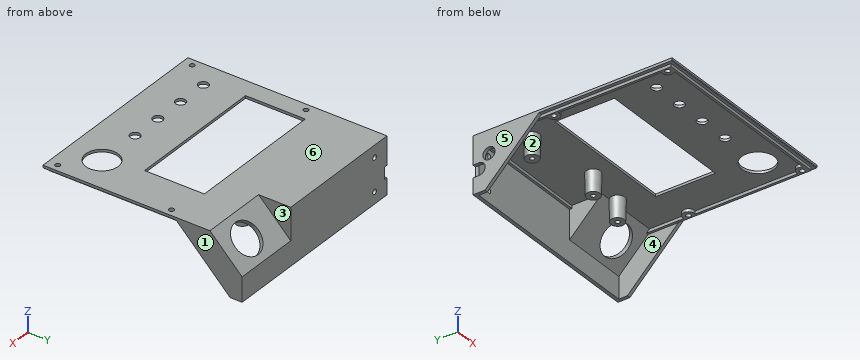
from build123d import *

# Parameters (mm, degrees)
CROQUIS1_W               = 140
CROQUIS1_H               = 140
FRENTE_DEPTH             = 1.8
CROQUIS32_W              = 135.2
CROQUIS32_H              = 135.2
CROQUIS32_W_2            = 132
CROQUIS32_H_2            = 132
SALIENTE_EXTRUIR5_DEPTH  = 2.1
SALIENTE_EXTRUIR6_DEPTH  = 2.1
VISERA_DEPTH             = 38
CORTAR_EXTRUIR1_DEPTH    = 2.4
SALIENTE_EXTRUIR9_DEPTH  = 50
CORTAR_EXTRUIR4_DEPTH    = 47
O_PE_REACH               = 113.138
CROQUIS39_R              = 11.25
CROQUIS15_R              = 1.75
ROSCA_DEPTH              = 3.9
MATRIZL1_COUNT           = 2
MATRIZL1_PITCH           = 80
MATRIZL1_COPY_1_DEPTH    = 2.1
MATRIZL1_COPY_2_SKETCH_R = 1.75
MATRIZL1_COPY_2_DEPTH    = 3.9
VISTA_DISPLAY_REACH      = 3.8
CROQUIS19_W              = 97.6
CROQUIS19_H              = 42
CROQUIS24_R              = 3.5
POTENCIOMETROS_DEPTH     = 1.8
MATRIZL3_COUNT           = 4
MATRIZL3_PITCH           = 22
CORTAR_EXTRUIR2_REACH    = 3.8
CROQUIS36_R              = 11.4
CHAFL_N1_SIZE            = 0.4
MPX_MOUNT_REACH          = 142
CROQUIS40_R              = 1.8
CROQUIS41_R              = 4.3
MPX_TUBBING_DEPTH        = 2.4
CROQUIS210_R             = 5
CROQUIS210_R_2           = 1.2
MEGA_UNO1_DEPTH          = 15
MEGA_UNO1_TAPER          = 1.5


with BuildPart() as part:
    # Croquis1 → FRENTE (new body)
    with BuildSketch(Plane.XY):
        Rectangle(CROQUIS1_W, CROQUIS1_H)
    extrude(amount=FRENTE_DEPTH)

    # Croquis32 → Saliente-Extruir5 (add)
    with BuildSketch(Plane(origin=(0, 0, 0), x_dir=(-1, 0, 0), z_dir=(0, 0, -1))):
        Rectangle(CROQUIS32_W, CROQUIS32_H)
        Rectangle(CROQUIS32_W_2, CROQUIS32_H_2, mode=Mode.SUBTRACT)
    extrude(amount=SALIENTE_EXTRUIR5_DEPTH)

    # Croquis33 → Saliente-Extruir6 (add)
    with BuildSketch(Plane(origin=(0, 0, 0), x_dir=(-1, 0, 0), z_dir=(0, 0, -1))):
        with BuildLine():
            Line((-67.6, -60.260263169), (-67.6, -66.339736831))
            ThreePointArc((-67.6, -66.339736831), (-61, -63.3), (-67.6, -60.260263169))
        make_face()
    saliente_extruir6 = extrude(amount=SALIENTE_EXTRUIR6_DEPTH)

    # Croquis29 → VISERA (add)
    with BuildSketch(Plane(origin=(0, 0, 0), x_dir=(-1, 0, 0), z_dir=(0, 0, -1))):
        Polygon((-70, 23.6), (-70, 70), (0, 70), (0, 67.6), (-67.6, 67.6), (-67.6, 23.6), align=None)
    visera = extrude(amount=VISERA_DEPTH)

    # Croquis30 → Cortar-Extruir1 (cut)
    with BuildSketch(Plane(origin=(70, 0, 0), x_dir=(0, 0, -1), z_dir=(1, 0, 0))):
        Polygon((0, 23.6), (38, 23.6), (38, 61.6), align=None)
    cortar_extruir1 = extrude(amount=-CORTAR_EXTRUIR1_DEPTH, mode=Mode.SUBTRACT)

    # Simetría3: VISERA, Cortar-Extruir1 across plane
    add(visera.mirror(Plane(origin=(0, 0, 0), x_dir=(0, 0, 1), z_dir=(1, 0, 0))))
    add(cortar_extruir1.mirror(Plane(origin=(0, 0, 0), x_dir=(0, 0, 1), z_dir=(1, 0, 0))), mode=Mode.SUBTRACT)

    # Croquis37 → Saliente-Extruir9 (add)
    with BuildSketch(Plane(origin=(70, 0, 0), x_dir=(0, 0, -1), z_dir=(1, 0, 0))):
        Polygon((25.070057685, 70), (-1.8, 43.129942315), (-1.8, 70), align=None)
    extrude(amount=-SALIENTE_EXTRUIR9_DEPTH)

    # Croquis38 → Cortar-Extruir4 (cut)
    with BuildSketch(Plane(origin=(70, 0, 0), x_dir=(0, 0, -1), z_dir=(1, 0, 0))):
        Polygon((20.827416998, 70), (-1.8, 47.372583002), (-1.8, 70), align=None)
    extrude(amount=-CORTAR_EXTRUIR4_DEPTH, mode=Mode.SUBTRACT)

    # Croquis39 → O-PE (cut, up to next)
    with BuildSketch(Plane(origin=(0, 24.586291501, 24.586291501), x_dir=(1, 0, 0), z_dir=(0, 0.707106781, 0.707106781)), mode=Mode.PRIVATE) as o_pe_sk1:
        with Locations((50, 48.224682477)):
            Circle(CROQUIS39_R)
    o_pe_tool1 = extrude(o_pe_sk1.sketch, amount=-O_PE_REACH, mode=Mode.PRIVATE) & part.part
    add(o_pe_tool1.solids().sort_by_distance((50, 58.686292, -9.513708))[0], mode=Mode.SUBTRACT)

    # Croquis15 → ROSCA (cut)
    with BuildSketch(Plane.XY.offset(1.8)):
        with Locations((65, -63.3)):
            Circle(CROQUIS15_R)
    rosca = extrude(amount=-ROSCA_DEPTH, mode=Mode.SUBTRACT)

    # Simetría4: Saliente-Extruir6, ROSCA across plane
    add(saliente_extruir6.mirror(Plane(origin=(0, 0, 0), x_dir=(0, 0, 1), z_dir=(1, 0, 0))))
    add(rosca.mirror(Plane(origin=(0, 0, 0), x_dir=(0, 0, 1), z_dir=(1, 0, 0))), mode=Mode.SUBTRACT)

    # MatrizL1: Saliente-Extruir6, ROSCA ×2
    with Locations(*[(0, i * MATRIZL1_PITCH, 0) for i in range(1, MATRIZL1_COUNT)]):
        add(saliente_extruir6)
        add(rosca, mode=Mode.SUBTRACT)

    # MatrizL1 copy 1 sketch → MatrizL1 copy 1 (add)
    with BuildSketch(Plane(origin=(0, 80, 0), x_dir=(1, 0, 0), z_dir=(0, 0, -1))):
        with BuildLine():
            Line((-67.6, 60.260263169), (-67.6, 66.339736831))
            ThreePointArc((-67.6, 66.339736831), (-61, 63.3), (-67.6, 60.260263169))
        make_face()
    extrude(amount=MATRIZL1_COPY_1_DEPTH)

    # MatrizL1 copy 2 sketch → MatrizL1 copy 2 (cut)
    with BuildSketch(Plane(origin=(0, 80, 1.8), x_dir=(-1, 0, 0), z_dir=(0, 0, 1))):
        with Locations((65, 63.3)):
            Circle(MATRIZL1_COPY_2_SKETCH_R)
    extrude(amount=-MATRIZL1_COPY_2_DEPTH, mode=Mode.SUBTRACT)

    # Croquis19 → VISTA-DISPLAY (cut, up to next)
    with BuildSketch(Plane(origin=(0, 0, 0), x_dir=(-1, 0, 0), z_dir=(0, 0, -1)), mode=Mode.PRIVATE) as vista_display_sk1:
        with Locations((8.2, 1)):
            Rectangle(CROQUIS19_W, CROQUIS19_H)
    vista_display_tool1 = extrude(vista_display_sk1.sketch, amount=-VISTA_DISPLAY_REACH, mode=Mode.PRIVATE) & part.part
    add(vista_display_tool1.solids().sort_by_distance((-8.2, 1, 0))[0], mode=Mode.SUBTRACT)

    # Croquis24 → POTENCIOMETROS (cut)
    with BuildSketch(Plane.XY.offset(1.8)):
        with Locations((-52, -46)):
            Circle(CROQUIS24_R)
    potenciometros = extrude(amount=-POTENCIOMETROS_DEPTH, mode=Mode.SUBTRACT)

    # MatrizL3: POTENCIOMETROS ×4
    with Locations(*[(i * MATRIZL3_PITCH, 0, 0) for i in range(1, MATRIZL3_COUNT)]):
        add(potenciometros, mode=Mode.SUBTRACT)

    # Croquis36 → Cortar-Extruir2 (cut, up to next)
    with BuildSketch(Plane(origin=(0, 0, 0), x_dir=(-1, 0, 0), z_dir=(0, 0, -1)), mode=Mode.PRIVATE) as cortar_extruir2_sk1:
        with Locations((-46, -46)):
            Circle(CROQUIS36_R)
    cortar_extruir2_tool1 = extrude(cortar_extruir2_sk1.sketch, amount=-CORTAR_EXTRUIR2_REACH, mode=Mode.PRIVATE) & part.part
    add(cortar_extruir2_tool1.solids().sort_by_distance((46, -46, 0))[0], mode=Mode.SUBTRACT)

    # Chaflán1
    chafl_n1_edges = [part.edges().sort_by_distance(p)[0] for p in [
        (0, -70, 0),
    ]]
    chamfer(chafl_n1_edges, length=CHAFL_N1_SIZE)

    # Croquis40 → MPX-MOUNT (cut, up to next)
    with BuildSketch(Plane(origin=(0, 70, 0), x_dir=(1, 0, 0), z_dir=(0, 1, 0)), mode=Mode.PRIVATE) as mpx_mount_sk1:
        with Locations((-58, 29.75)):
            Circle(CROQUIS40_R)
    mpx_mount_tool1 = extrude(mpx_mount_sk1.sketch, amount=-MPX_MOUNT_REACH, mode=Mode.PRIVATE) & part.part
    add(mpx_mount_tool1.solids().sort_by_distance((-58, 70, -29.75))[0], mode=Mode.SUBTRACT)
    # Croquis40 → MPX-MOUNT (cut, up to next)
    with BuildSketch(Plane(origin=(0, 70, 0), x_dir=(1, 0, 0), z_dir=(0, 1, 0)), mode=Mode.PRIVATE) as mpx_mount_sk2:
        with Locations((-58, 6.65)):
            Circle(CROQUIS40_R)
    mpx_mount_tool2 = extrude(mpx_mount_sk2.sketch, amount=-MPX_MOUNT_REACH, mode=Mode.PRIVATE) & part.part
    add(mpx_mount_tool2.solids().sort_by_distance((-58, 70, -6.65))[0], mode=Mode.SUBTRACT)

    # Croquis41 → MPX-TUBBING (cut)
    with BuildSketch(Plane.ZY.offset(70)):
        with Locations((-14.13, 58.78)):
            Circle(CROQUIS41_R)
        with BuildLine():
            Line((-26.56, 70), (-26.56, 65.74))
            ThreePointArc((-26.56, 65.74), (-22.26, 61.44), (-17.96, 65.74))
            Line((-17.96, 65.74), (-17.96, 70))
            Line((-17.96, 70), (-26.56, 70))
        make_face()
    extrude(amount=-MPX_TUBBING_DEPTH, mode=Mode.SUBTRACT)

    # Croquis210 → Mega-UNO1 (add)
    with BuildSketch(Plane(origin=(-7.163025125, 18.178552878, 0), x_dir=(-1, 0, 0), z_dir=(0, 0, -1))):
        with Locations((44.866974875, 23.281447122)):
            Circle(CROQUIS210_R)
        with Locations((44.866974875, 23.281447122)):
            Circle(CROQUIS210_R_2, mode=Mode.SUBTRACT)
        with Locations((-7.203025125, 18.201447122)):
            Circle(CROQUIS210_R)
        with Locations((-7.203025125, 18.201447122)):
            Circle(CROQUIS210_R_2, mode=Mode.SUBTRACT)
        with Locations((-37.683025125, 23.281447122)):
            Circle(CROQUIS210_R)
        with Locations((-37.683025125, 23.281447122)):
            Circle(CROQUIS210_R_2, mode=Mode.SUBTRACT)
    extrude(amount=MEGA_UNO1_DEPTH, taper=MEGA_UNO1_TAPER)


solid = part.part
Design review of the part built by this model. Coordinates are the model's own, in mm. Face numbers are marked on the shaded views. A direction names the side the tool comes from. Give positions to 0.01 mm unless a question says otherwise; leave off trailing zeros. Write each loop counter-clockwise with the first axis right and the second up, starting at its lowest first coordinate (ties: lowest second). Pieces come first, ordered by that corner, then holes. Notation, with made-up numbers: M -11.75,-16 L 42.25,-16 A31 ccw 42.25,8 Z; hole C 30,18 d2. An arc over 180 degrees is marked long. Answer as a JSON object with one key per item and string values. Group by question number.
1) We need section A-A (y = -63.3). Give the boundary of the cut face in (x, z), and give its area (3 significant figures).
2) Clearance check with flat-ended pins moving along their axes: pin 1 Ø12 at (x, z) = (-43, -7.5) entering from -Y; pin 2 Ø1.1 at (y, z) = (-26, -0.5) entering from +X; pin 3 Ø12 at (y, z) = (-44.5, -7.5) entering from -X; pin 4 Ø6 at (x, z) = (-58, -6.65) entering from -Y. State where each tip first meets the part, or that it passes through.
3) Tool access review of the marked faces 1, 2 and 3: name each direction out of +Z, -Z, +X, -X, +Y, -Y from which nothing blocks a thin tool from reaching the whole face with its end or side.
4) Mouldability with a two-part tool opening along X and no side actions: class the marked faces 4, 5 and 6 as released by +X, released by -X, zero draft, split by the parting line, or undercut.
5) We need section B-B (x = -22.5). Give the boundary of the cut face in (y, z), and give its area (3 significant figures).
6) We need section C-C (z = -29.75). Give the boundary of the cut face in (x, y), and give its area (3 significant figures).
7) For line 1 along Y through (x, z) = (-31, -2); line 2 along X through (y, z) = (64, -36); line 3 along Y through (x, z) = (65, -1), list the stretches that pass through material, from the lowest coordinate up.
8) We need section D-D (y = -37.5). Give the boundary of the cut face in (x, z), and give its area (3 significant figures).
Answer key:
{
 "1": {"outline": "M -70,0 L -67.6,0 L -67.6,-2.1 L -66.75,-2.1 L -66.75,1.8 L -70,1.8 Z; M -63.25,-2.1 L -61,-2.1 L -61,0 L 61,0 L 61,-2.1 L 63.25,-2.1 L 63.25,1.8 L -63.25,1.8 Z; M 66.75,-2.1 L 67.6,-2.1 L 67.6,0 L 70,0 L 70,1.8 L 66.75,1.8 Z", "area": "252 mm²"},
 "2": {"pin 1": "stops at y = -67.6", "pin 2": "stops at x = 70", "pin 3": "stops at x = -67.6", "pin 4": "stops at y = 37.65"},
 "3": {"face 1": "+Z, -Z, +X, +Y, -Y", "face 2": "-Z", "face 3": "+Z, +X, +Y"},
 "4": {"face 4": "undercut", "face 5": "released by -X", "face 6": "zero draft"},
 "5": {"outline": "M -70,0.4 L -69.6,0 L -67.6,0 L -67.6,-2.1 L -66,-2.1 L -66,0 L -20,0 L -20,1.8 L -70,1.8 Z; M 22,0 L 66,0 L 66,-2.1 L 67.6,-2.1 L 67.6,-38 L 70,-38 L 70,1.8 L 22,1.8 Z", "area": "274 mm²"},
 "6": {"outline": "M -70,53.35 L -67.6,53.35 L -67.6,67.6 L -59.8,67.6 L -59.8,70 L -70,70 Z; M -56.2,67.6 L 67.6,67.6 L 67.6,53.35 L 70,53.35 L 70,70 L -56.2,70 Z", "area": "396 mm²"},
 "7": {"line 1": "y = -67.6 to -66, 66 to 70", "line 2": "x = -70 to -67.6, 67.6 to 70", "line 3": "y = -67.6 to -65.05, -61.55 to -59.3, 12.7 to 14.95, 18.45 to 20.7, 45.93 to 50.17"},
 "8": {"outline": "M -70,0 L -67.6,0 L -67.6,-2.1 L -66,-2.1 L -66,0 L 38.4,0 L 38.4,1.8 L -70,1.8 Z; M 53.6,0 L 66,0 L 66,-2.1 L 67.6,-2.1 L 67.6,0 L 70,0 L 70,1.8 L 53.6,1.8 Z", "area": "231 mm²"}
}
